Can you work these out from the drawing? Everything is in mm from the part's minimum corner. Give positions to 0.01 mm unless a question says otherwise; leave off trailing zeros. Order: outer loops, then holes, each group sorted by start corner. A loop starts at its lowest first (then second) coordinate and runs counter-clockwise, first axis right, second up. Notation, with made-up numbers: (60.25, 86) -> (92.25, 86) arc R29 cw to (92.25, 125) -> close; hole circle Ø10 at (-27.75, 47.25). An arc over 180 degrees is marked (long way). One line per item, written item: value.
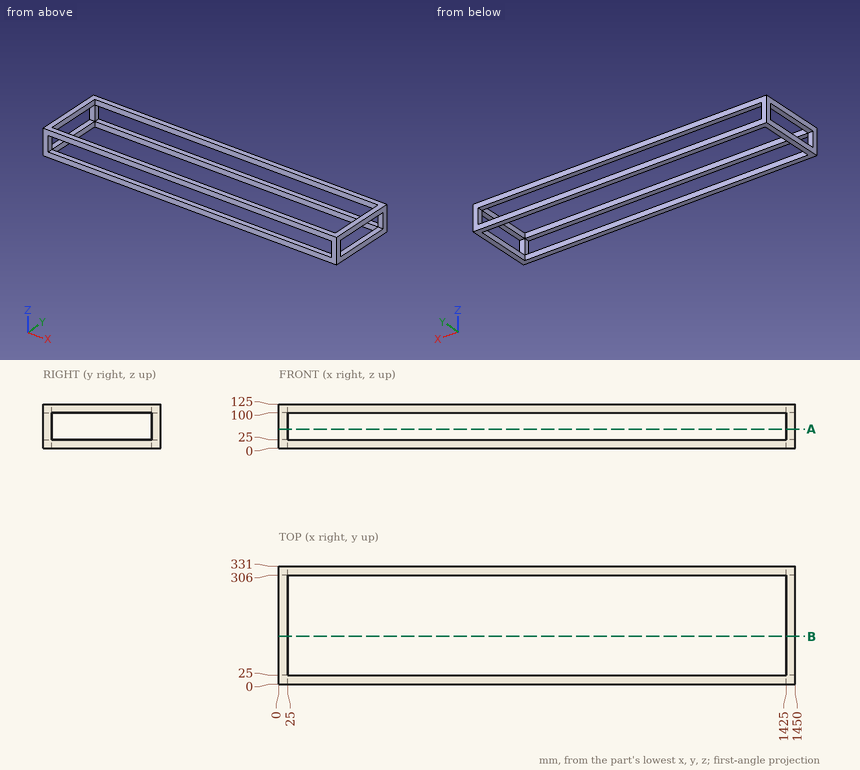
1) Suppose I cut it at B-B, the plane y = 135. Write out the boundary of the cut face in (x, z), then the cut area to 3 significant figures.
Answer below:
outline: (0, 0) -> (25, 0) -> (25, 25) -> (0, 25) -> close; (0, 100) -> (25, 100) -> (25, 125) -> (0, 125) -> close; (1425, 0) -> (1450, 0) -> (1450, 25) -> (1425, 25) -> close; (1425, 100) -> (1450, 100) -> (1450, 125) -> (1425, 125) -> close
area: 2,500 mm2
2) For P1, Ø5, axis at x = 557, z = 98.5, coming from the +Y side, with a flat end and sliding along its axis, tell me the tip position at first contact or that it passes through.
Answer below:
P1: stops at y = 331
3) If I drill on line 1 along X through (y, z) = (214.5, 117.5); line 2 along Y through (x, z) = (794.5, 115), over which ranges is the centre line in solid material (lowest first)?
Answer below:
line 1: x = 0 to 25, 1425 to 1450
line 2: y = 0 to 25, 306 to 331
4) Suppose I cut it at A-A, the plane z = 54.5. Write out the boundary of the cut face in (x, y), then the cut area to 3 significant figures.
Answer below:
outline: (0, 0) -> (25, 0) -> (25, 25) -> (0, 25) -> close; (0, 306) -> (25, 306) -> (25, 331) -> (0, 331) -> close; (1425, 0) -> (1450, 0) -> (1450, 25) -> (1425, 25) -> close; (1425, 306) -> (1450, 306) -> (1450, 331) -> (1425, 331) -> close
area: 2,500 mm2
